Solid Edge part; units mm, degrees
sketch "Sketch1" plane through (0, 0, 0) normal (0, 0, 1) x (1, 0, 0)
  line L0 (400, 250) -> (-400, 250)
  line L1 (-400, 150) -> (-400, 250)
  line L2 (-50, 0) -> (-400, 150)
  arc A0 (50, 0) -> (-50, 0) centre (0, 0) cw
  line L3 (50, 0) -> (400, 150)
  line L4 (400, 150) -> (400, 250)
extrude "Protrusion1" add sketch "Sketch1" against normal blind 20
hole "Bohrung_1" at (0, 0, 0) direction (0, 0, -1) diameter 40 end up to next
hole "Bohrung_2" at (0, 0, 0) direction (0, 0, -1) diameter 52 depth 5
hole "Bohrung_3" at (-380, 230, 0) direction (0, 0, -1) diameter 8.376 end up to next start chamfer 1 start chamfer angle 45
hole "Hole1" at (-380, 170, 0) direction (0, 0, -1) diameter 8.376 end up to next start chamfer 1 start chamfer angle 45
hole "Hole2" at (380, 170, 0) direction (0, 0, -1) diameter 8.376 end up to next start chamfer 1 start chamfer angle 45
hole "Hole3" at (380, 230, 0) direction (0, 0, -1) diameter 8.376 end up to next start chamfer 1 start chamfer angle 45
The model under review builds one solid part; all positions refer to its coordinate system, in mm. A direction names the side the tool comes from. Round coordinates to 2 decimals unless told otherwise and drop trailing zeros. Order: outer loops, then holes, each group sorted by start corner. A loop starts at its lowest first (then second) coordinate and runs counter-clockwise, first axis right, second up. Notation, with made-up numbers: (6.25, 3) -> (31.25, 3) arc R9 cw to (31.25, 8) -> close; hole circle Ø9 at (-19, -6.5). An arc over 180 degrees is marked (long way). Use a Markdown table: item, result.
Q1. We need section B-B on z = -17. Write out the cut boundary in (x, y), then the cut area to 3 significant figures.
Values:
| item | result |
|---|---|
| outline | (-400, 150) -> (-50, 0) arc R50 ccw to (50, 0) -> (400, 150) -> (400, 250) -> (-400, 250) -> close; hole circle Ø8.38 at (-380, 170); hole circle Ø8.38 at (-380, 230); hole circle Ø40 at (0, 0); hole circle Ø8.38 at (380, 170); hole circle Ø8.38 at (380, 230) |
| area | 150,000 mm^2 |
Q2. Tool access review of faces 1 (the cylindrical face through (15.821, 20.633, -2.535)), 2 (the flat face through (222.55, 73.95, -9.86)): name each direction out of +Z, -Z, +X, -X, +Y, -Y from which nothing blocks a thin tool from reaching the whole face with its end or side.
Values:
| item | result |
|---|---|
| face 1 | +Z |
| face 2 | +Z, -Z, +X, -Y |
Q3. We need section D-D on y = 132. Write out the cut boundary in (x, z).
Values:
| item | result |
|---|---|
| outline | (-358, -20) -> (358, -20) -> (358, 0) -> (-358, 0) -> close |
Q4. For line 1 (X direction, y = 230, z = -14.75); line 2 (Y direction, x = -380, z = -13.5); line 3 (Y direction, x = 341, z = -9.25), list the stretches that pass through material, from the lowest coordinate up.
Values:
| item | result |
|---|---|
| line 1 | x = -400 to -384.19, -375.81 to 375.81, 384.19 to 400 |
| line 2 | y = 141.43 to 165.81, 174.19 to 225.81, 234.19 to 250 |
| line 3 | y = 124.71 to 250 |
Q5. Mouldability with a two-part tool opening along Y and no side actions: class faces 3 (the flat face through (6, 250, -10)), 4 (the cylindrical face through (-1.099, -49.988, -9.86)), 5 (the cylindrical face through (-19.524, 4.336, -12.395)) as +Y half, -Y half, draft (parallel to the pull), parting line (faces both ways), or undercut.
Values:
| item | result |
|---|---|
| face 3 | +Y half |
| face 4 | -Y half |
| face 5 | undercut |
Q6. Clearance check with flat-ended pins moving along their axes: P1, Ø5, axis at x = 380, y = 230, coming from the -Z side; P2, Ø4, axis at y = -8.5, z = -17, coming from the -X side; P3, Ø1.5, axis at y = 54.5, z = -11, coming from the +X side; P4, Ø4, axis at x = -169.5, z = -2, coming from the -Y side. State where each tip first meets the part, or that it passes through.
Values:
| item | result |
|---|---|
| P1 | passes through |
| P2 | stops at x = -49.58 |
| P3 | stops at x = 178.92 |
| P4 | stops at y = 50.36 |
Q7. We need section A-A on x = 0. Write out the cut boundary in (y, z), then the cut area to 3 significant figures.
Values:
| item | result |
|---|---|
| outline | (-50, -20) -> (-20, -20) -> (-20, -5) -> (-26, -5) -> (-26, 0) -> (-50, 0) -> close; (20, -20) -> (250, -20) -> (250, 0) -> (26, 0) -> (26, -5) -> (20, -5) -> close |
| area | 5,140 mm^2 |
Q8. We need section C-C on y = 9.5. Write out the cut boundary in (x, z), then the cut area to 3 significant figures.
Values:
| item | result |
|---|---|
| outline | (-72.17, -20) -> (-17.6, -20) -> (-17.6, -5) -> (-24.2, -5) -> (-24.2, 0) -> (-72.17, 0) -> close; (17.6, -20) -> (72.17, -20) -> (72.17, 0) -> (24.2, 0) -> (24.2, -5) -> (17.6, -5) -> close |
| area | 2,120 mm^2 |
